The listing builds one solid part. Answer for the finished solid, in the listing's coordinates (mm). A direction names the side the tool comes from. Round coordinates to 2 decimals unless told otherwise and drop trailing zeros. Write each loop counter-clockwise with the first axis right and the second up, starting at its lowest first coordinate (ties: lowest second). Pieces come first, ordered by that corner, then holes. Notation, with made-up numbers: (14, -39.5) - (29, -39.5) arc R12 ccw to (29, -29.5) - close; hole circle Ø1 at (50, 8.5). An arc over 180 degrees is marked (long way). Answer in a Markdown table with one row per item.
from build123d import *

# Parameters (mm, degrees)
SKETCH_1_R          = 19
EXTRUDE_1_DEPTH     = 31
SKETCH_2_R          = 8
EXTRUDE_2_DEPTH     = 7
SKETCH_3_R          = 3
CUT_EXTRUDE_1_DEPTH = 47.540305113
SKETCH_4_R          = 12
EXTRUDE_3_DEPTH     = 2
SKETCH_5_R          = 10
SKETCH_5_R_2        = 3
EXTRUDE_4_DEPTH     = 1


with BuildPart() as part:
    # 草图1 → 凸台-拉伸1 (new body)
    with BuildSketch(Plane.XY):
        Circle(SKETCH_1_R)
    extrude(amount=EXTRUDE_1_DEPTH)

    # 草图2 → 凸台-拉伸2 (add)
    with BuildSketch(Plane.XY.offset(31)):
        Circle(SKETCH_2_R)
    extrude(amount=EXTRUDE_2_DEPTH)

    # 草图3 → 切除-拉伸1 (cut, through all)
    with BuildSketch(Plane.XY.offset(38)):
        Circle(SKETCH_3_R)
    extrude(amount=-CUT_EXTRUDE_1_DEPTH, mode=Mode.SUBTRACT)

    # 草图4 → 凸台-拉伸3 (add)
    with BuildSketch(Plane.XY.offset(31)):
        Circle(SKETCH_4_R)
    extrude(amount=EXTRUDE_3_DEPTH)

    # 草图5 → 凸台-拉伸4 (add)
    with BuildSketch(Plane(origin=(0, 0, 0), x_dir=(-1, 0, 0), z_dir=(0, 0, -1))):
        with Locations(Location((0, 0, 0), (0, 0, 180))):
            Circle(SKETCH_5_R)
        with Locations(Location((0, 0, 0), (0, 0, 180))):
            Circle(SKETCH_5_R_2, mode=Mode.SUBTRACT)
    extrude(amount=EXTRUDE_4_DEPTH)


solid = part.part
(1) Find the intervals of material crossed by line 1 (Z direction, x = 10, y = -10.5); line 2 (Y direction, x = 0, z = 35.1); line 3 (Z direction, x = -1.5, y = 9), in increasing order.
Checked values:
| item | result |
|---|---|
| line 1 | z = 0 to 31 |
| line 2 | y = -8 to -3, 3 to 8 |
| line 3 | z = -1 to 33 |
(2) Section A-A (x = 0) is taken. Give the vertices of the cut face in (y, z).
Checked values:
| item | result |
|---|---|
| outline | (-19, 0) - (-10, 0) - (-10, -1) - (-3, -1) - (-3, 31) - (3, 31) - (3, -1) - (10, -1) - (10, 0) - (19, 0) - (19, 31) - (12, 31) - (12, 33) - (8, 33) - (8, 38) - (3, 38) - (3, 33) - (-3, 33) - (-3, 38) - (-8, 38) - (-8, 33) - (-12, 33) - (-12, 31) - (-19, 31) - close |
(3) Flat-ended cylindrical pins translate along their axes: pin 1 (1.5 mm diameter, centred on x = -12.5, y = 13.5, fed in from +Z); pin 2 (5 mm diameter, centred on x = 5, z = 23.5, fed in from +Y); pin 3 (8 mm diameter, centred on x = 11.5, y = -12.5, fed in from -Z). Find the tip coordinate at first contact, or state that the pin passes through.
Checked values:
| item | result |
|---|---|
| pin 1 | stops at z = 31 |
| pin 2 | stops at y = 18.83 |
| pin 3 | stops at z = 0 |
(4) Section D-D (x = -11) is taken. Give the vertices of the cut face in (y, z).
Checked values:
| item | result |
|---|---|
| outline | (-15.49, 0) - (15.49, 0) - (15.49, 31) - (4.8, 31) - (4.8, 33) - (-4.8, 33) - (-4.8, 31) - (-15.49, 31) - close |
(5) For a pull along X with two mould halves and no side action, classify faces 4 (the flat face through (-0.3, -12.4, 31)), 5 (the cylindrical face through (-11.99, 0.53, 31.99)), 6 (the cylindrical face through (-3, 0, 36)) as pulls with the +X half, pulls with the -X half, needs draft (parallel to the pull), parting line crosses it, or undercut.
Checked values:
| item | result |
|---|---|
| face 4 | needs draft |
| face 5 | parting line crosses it |
| face 6 | undercut |
(6) Section C-C (z = 2.5) is taken. Give the vertices of the cut face in (x, y).
Checked values:
| item | result |
|---|---|
| outline | circle Ø38 at (0, 0); hole circle Ø6 at (0, 0) |
(7) For faces 1 (the flat face through (3.4, 0.1, 38)), 2 (the flat face through (0, 0, 31)), 3 (the flat face through (2, -8, 33)), determine the directions among +Z, -Z, +X, -X, +Y, -Y from which every point of the face is accessible in a straight line to the end or side of a thin tool.
Checked values:
| item | result |
|---|---|
| face 1 | +Z, +X, -X, +Y, -Y |
| face 2 | -Z |
| face 3 | +Z |
